Design review of the part built by this model. Coordinates are the model's own, in mm. A direction names the side the tool comes from. Round coordinates to 2 decimals unless told otherwise and drop trailing zeros. Loops run counter-clockwise (first coordinate to the right, second up) from the corner with the lowest first, then second, coordinate; pieces in that order, holes last. Notation, with made-up numbers: (61.25, 1) - (100.25, 1) arc R34 cw to (100.25, 39) - close; hole circle Ø10 at (9, 86). An arc over 180 degrees is marked (long way). Answer as CSV lines item,"result". Start each with the question number.
(1) Consider section D-D (z = 14). Give the boundary of the cut face in (x, y).
(2) Wall thickness on L1, parallel to X at y = 106.5, z = 26.75; L2, parallel to Y at x = -69.5, z = 32.5; L3, parallel to Z at x = -60, y = 110.5: over which ranges is each line inside the solid? List them lowest first.
(3) Consider section C-C (x = -60). Give the boundary of the cut face in (y, z).
(4) Consider section A-A (z = 26.75). Give the boundary of the cut face in (x, y), and give its area (3 significant figures).
(5) Consider section B-B (y = 109.75). Give the boundary of the cut face in (x, z), and give its area (3 significant figures).
(6) For faces 1 (the cylindrical face through (-59.9, 97.8, 23.7)), 2 (the flat face through (-23, 115.72, 12)), 3 (the flat face through (-23, 98.155, 60)), 4 (the flat face through (-70, 94.8, 26)), 5 (the flat face through (-52, 100.62, 26)), list the 3-axis set-ups (+Z, -Z, +X, -X, +Y, -Y) from which the entire face can be reached by the end or side of a thin tool; tool diameter is ignored.
(7) For P1, Ø6, axis at x = -24.5, y = 98.5, coming from the +Z side; P2, Ø2, axis at y = 108, z = 15.5, coming from the -X side; P3, Ø8, axis at x = -81.5, y = 111, coming from the +Z side, all flat-tipped, find the tip position at first contact; note any pin that passes through.
(8) Mouldability with a two-part tool opening along Z and no side actions: class faces 6 (the cylindrical face through (-59.8, 97.8, 29.8)), 7 (the flat face through (-97, 112.365, 60)), 8 (the cylindrical face through (-14.644, 105.359, 45.556)) as released by +Z, released by -Z, zero draft, split by the parting line, or undercut.
from build123d import *

# Parameters (mm, degrees)
EXTRUDE198_DEPTH           = 40
EXTRUDE198_ROLL_ANGLE      = -90
EXTRUDE198_PLACEMENT_ANGLE = 90
SKETCH181_R                = 39.566192
EXTRUDE197_DEPTH           = 20
CUT124_PLACEMENT_ANGLE     = 270


with BuildPart() as pieza_clave_motor011:
    # Sketch182 → Extrude198 (new body)
    with BuildSketch(Plane(origin=(0, -17.4, 11), x_dir=(-1, 0, 0), z_dir=(0, 1, 0))):
        with BuildLine():
            Line((-2.055, -8.921835), (2.055, -8.921835))
            ThreePointArc((2.055, -13.431835), (3.05091, -11.176835), (2.055, -8.921835))
            Line((2.055, -13.431835), (-2.055, -13.431835))
            ThreePointArc((-2.055, -8.921835), (-3.05091, -11.176835), (-2.055, -13.431835))
        make_face()
    extrude(amount=EXTRUDE198_DEPTH)


with BuildPart() as pieza_clave_motor011_1:
    # Extrude198 roll: moved
    add(pieza_clave_motor011.part.rotate(Axis((0, 0, 0), (1, 0, 0)), EXTRUDE198_ROLL_ANGLE))


with BuildPart() as pieza_clave_motor011_2:
    # Extrude198 placement: moved
    add(pieza_clave_motor011_1.part.moved(Location((0, 0, 13.85))).rotate(Axis((0, 0, 13.85), (0, 0, 1)), EXTRUDE198_PLACEMENT_ANGLE))


with BuildPart() as extrude197:
    # Sketch181 (on Face7 of Revolve004) → Extrude197 (new body)
    with BuildSketch(Plane.XY.offset(20.92)):
        Circle(SKETCH181_R)
    extrude(amount=EXTRUDE197_DEPTH)


with BuildPart() as extrude197_1:
    # Extrude197 placement: moved
    add(extrude197.part.moved(Location((0, 0, -15.1))))


with BuildPart() as obj1:
    # Sketch180 → Revolve004 (revolve)
    with BuildSketch(Plane.XZ):
        Polygon((0, 0), (50.12, 0), (50.12, 3.355495), (49.1, 3.355495), (49.1, 17.564505), (50.12, 17.564505), (50.12, 20.92), (0, 20.92), align=None)
    revolve(axis=Axis((0, 0, 0), (0, 0, 1)))

    # Cut125: cut Extrude197
    add(extrude197_1.part, mode=Mode.SUBTRACT)

    # Cut124: cut Pieza Clave motor011
    add(pieza_clave_motor011_2.part, mode=Mode.SUBTRACT)


with BuildPart() as obj1_1:
    # Cut124 placement: moved
    add(obj1.part.moved(Location((-60, 94.8, 26.75))).rotate(Axis((-60, 94.8, 26.75), (1, 0, 0)), CUT124_PLACEMENT_ANGLE))


solid = obj1_1.part
Determined:
1,outline,"(-108.47, 94.8) - (-11.53, 94.8) - (-11.53, 98.16) - (-12.58, 98.16) - (-12.58, 112.36) - (-11.53, 112.36) - (-11.53, 115.72) - (-22.54, 115.72) - (-22.54, 100.62) - (-97.46, 100.62) - (-97.46, 115.72) - (-108.47, 115.72) - (-108.47, 112.36) - (-107.42, 112.36) - (-107.42, 98.16) - (-108.47, 98.16) - close"
2,L1,"x = -109.1 to -99.57, -20.43 to -10.9"
2,L2,"y = 94.8 to 100.62"
2,L3,"z = -22.35 to -12.82, 66.32 to 75.85"
3,outline,"(94.8, -23.37) - (98.16, -23.37) - (98.16, -22.35) - (112.36, -22.35) - (112.36, -23.37) - (115.72, -23.37) - (115.72, -12.82) - (100.62, -12.82) - (100.62, 23.7) - (94.8, 23.7) - close; (94.8, 29.8) - (100.62, 29.8) - (100.62, 66.32) - (115.72, 66.32) - (115.72, 76.87) - (112.36, 76.87) - (112.36, 75.85) - (98.16, 75.85) - (98.16, 76.87) - (94.8, 76.87) - close"
4,outline,"(-110.12, 94.8) - (-62.08, 94.8) - (-62.08, 100.62) - (-99.57, 100.62) - (-99.57, 115.72) - (-110.12, 115.72) - (-110.12, 112.36) - (-109.1, 112.36) - (-109.1, 98.16) - (-110.12, 98.16) - close; (-57.57, 94.8) - (-9.88, 94.8) - (-9.88, 98.16) - (-10.9, 98.16) - (-10.9, 112.36) - (-9.88, 112.36) - (-9.88, 115.72) - (-20.43, 115.72) - (-20.43, 100.62) - (-57.57, 100.62) - close"
4,area,"847 mm^2"
5,outline,"circle Ø98.2 at (-60, 26.75); hole circle Ø79.13 at (-60, 26.75)"
5,area,"2,660 mm^2"
6,face 1,"+Y, -Y"
6,face 2,"+Z, -Z, +X, -X, +Y"
6,face 3,"none"
6,face 4,"+Z, -Z, +X, -X, -Y"
6,face 5,"+Y"
7,P1,"stops at z = 64.89"
7,P2,"stops at x = -108.02"
7,P3,"stops at z = 73.63"
8,face 6,"undercut"
8,face 7,"zero draft"
8,face 8,"split by the parting line"
